from build123d import *

# Parameters (mm, degrees)
SKETCH1_W               = 67.31
SKETCH1_H               = 88.9
EXTRUDE1_DEPTH          = 12.7
SKETCH2_R               = 18.1356
EXTRUDE2_DEPTH          = 58.181741185
SKETCH3_W               = 28.468633454
SKETCH3_H               = 1.016
EXTRUDE3_DEPTH          = 58.181741185
F_1_4_CLEARANCE_HOLE1_D = 6.7564
SKETCH10_W              = 15.24
SKETCH10_H              = 31.75
EXTRUDE4_DEPTH          = 58.181741185
FILLET1_R               = 2.54
FILLET1_OF_MIRROR2_R    = 2.54


with BuildPart() as part:
    # Sketch1 → Extrude1 (new body)
    with BuildSketch(Plane.XY):
        Rectangle(SKETCH1_W, SKETCH1_H)
    extrude(amount=EXTRUDE1_DEPTH)

    # Sketch2 → Extrude2 (cut, through all)
    with BuildSketch(Plane.XY.offset(12.7)):
        with Locations((-9.525, 0)):
            Circle(SKETCH2_R)
    extrude(amount=-EXTRUDE2_DEPTH, mode=Mode.SUBTRACT)

    # Sketch3 → Extrude3 (cut, through all)
    with BuildSketch(Plane.XY.offset(12.7)):
        with Locations((21.1328, 0)):
            Rectangle(SKETCH3_W, SKETCH3_H)
    extrude(amount=-EXTRUDE3_DEPTH, mode=Mode.SUBTRACT)

    # 1/4 Clearance Hole1 (through all)
    with Locations(Plane(origin=(27.305, 44.45, 6.35), x_dir=(0, 0, 1), z_dir=(0, 1, 0))):
        with Locations((0, 0)):
            Hole(F_1_4_CLEARANCE_HOLE1_D / 2)

    # Sketch9 → CSK for 1/2 Flat Head Machine Screw (100)1 (revolve, cut)
    with BuildSketch(Plane(origin=(-20.955, 31.75, 12.7), x_dir=(0, -1, 0), z_dir=(1, 0, 0))):
        Polygon((0, 0), (0, 15.483549943), (6.74624, 11.43), (6.74624, 5.17695943), (12.9159, 0), align=None)
    csk_for_1_2_flat_head_machine_screw_100 = revolve(axis=Axis((-20.955, 31.75, 19.05), (0, 0, -1)), mode=Mode.SUBTRACT)

    # Mirror1: CSK for 1/2 Flat Head Machine Screw (100)1 across plane
    add(csk_for_1_2_flat_head_machine_screw_100.mirror(Plane.ZX), mode=Mode.SUBTRACT)

    # Sketch10 → Extrude4 (cut, through all)
    with BuildSketch(Plane.XY.offset(12.7)):
        with Locations((26.035, 28.575)):
            Rectangle(SKETCH10_W, SKETCH10_H)
    extrude4 = extrude(amount=-EXTRUDE4_DEPTH, mode=Mode.SUBTRACT)

    # Fillet1
    fillet1_edges = [part.edges().sort_by_distance(p)[0] for p in [
        (18.415, 12.7, 6.35),
    ]]
    fillet(fillet1_edges, radius=FILLET1_R)

    # Mirror2: Extrude4 across plane
    add(extrude4.mirror(Plane.ZX), mode=Mode.SUBTRACT)

    # Fillet1 of Mirror2
    fillet1_of_mirror2_edges = [part.edges().sort_by_distance(p)[0] for p in [
        (18.415, -12.7, 6.35),
    ]]
    fillet(fillet1_of_mirror2_edges, radius=FILLET1_OF_MIRROR2_R)


solid = part.part
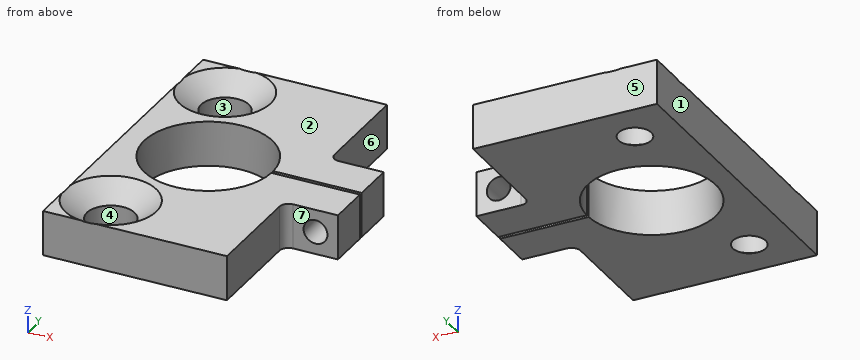
The model under review builds one solid part; all positions refer to its coordinate system, in mm. Face numbers are marked on the shaded views. A direction names the side the tool comes from. Round coordinates to 2 decimals unless told otherwise and drop trailing zeros. Write each loop counter-clockwise with the first axis right and the second up, starting at its lowest first coordinate (ties: lowest second). Pieces come first, ordered by that corner, then holes. Notation, with made-up numbers: M 20.25,37 L 71.25,37 A25 ccw 71.25,60 Z; hole C -2.5,35 d5. An arc over 180 degrees is marked long. Answer as CSV lines item,"result". Start each with the question number.
Q1. Tool access review of the marked faces 4, 5, 6 and 7: name each direction out of +Z, -Z, +X, -X, +Y, -Y from which nothing blocks a thin tool from reaching the whole face with its end or side.
Q2. Clearance check with flat-ended pins moving along their axes: P1, Ø11, axis at x = -20.955, y = -31.75, coming from the +Z side; P2, Ø12, axis at x = 21, y = -21.5, coming from the +Z side; P3, Ø6.5, axis at x = 28.5, z = 4.5, coming from the +Y side; P4, Ø4, axis at y = 25.5, z = 9, coming from the +X side (3 decimals). State where each tip first meets the part, or that it passes through.
Q3. Consider section A-A, the plane z = 5.75. State how many separate pieces and enclosed holes the cut face has, then the cut area to 3 significant figures.
Q4. Consider section C-C, the plane x = -3. Give the boundary of the cut face in (y, z), then the cut area to 3 significant figures.
Q5. The part is to be moulded in two halves that separate along X. For the marked faces 1, 2 and 3, say which applies: +X half, -X half, draft (parallel to the pull), parting line (faces both ways), or undercut.
Q6. Wall thickness on line 1 along Y through (x, z) = (13, 4.5); line 2 along X through (y, z) = (-6, 6.35) (3 decimals); line 3 along X through (y, z) = (31.75, 6.25) (3 decimals): over which ranges is each line inside the solid? List them lowest first.
Q7. Consider section B-B, the plane y = 31.75. Give the boundary of the cut face in (x, z) (3 decimals), then the cut area to 3 significant figures.
Q8. Consider section D-D, the plane y = -2. Give the boundary of the cut face in (x, z) (3 decimals).
Result set:
1,face 4,"+Z"
1,face 5,"+Z, -Z, +X, -X, +Y"
1,face 6,"+Z, -Z, +X, +Y"
1,face 7,"+Z, -Z, +X, -Y"
2,P1,"stops at z = 0.52"
2,P2,"stops at z = 12.7"
2,P3,"stops at y = 12.7"
2,P4,"stops at x = 18.415"
3,separate pieces,"3"
3,enclosed holes,"2"
3,area,"3,510 mm²"
4,outline,"M -44.45,0 L -16.92,0 L -16.92,12.7 L -44.45,12.7 Z; M 16.92,0 L 44.45,0 L 44.45,12.7 L 16.92,12.7 Z"
4,area,"699 mm²"
5,face 1,"-X half"
5,face 2,"draft"
5,face 3,"undercut"
6,line 1,"y = -44.45 to -0.51, 0.51 to 44.45"
6,line 2,"x = -33.655 to -26.639, 7.589 to 23.927, 30.683 to 33.655"
6,line 3,"x = -33.655 to -27.701, -14.209 to 18.415"
7,outline,"M -33.655,0 L -25.588,0 L -27.701,1.27 L -27.701,7.523 L -33.655,12.519 Z; M -16.322,0 L 18.415,0 L 18.415,12.7 L -8.039,12.7 L -14.209,7.523 L -14.209,1.27 Z"
7,area,"461 mm²"
8,outline,"M -33.655,0 L -27.55,0 L -27.55,12.7 L -33.655,12.7 Z; M 8.5,0 L 33.655,0 L 33.655,12.7 L 8.5,12.7 Z; hole C 27.305,6.35 d6.756"
